Verification items for the finished model (mm, model axes). A direction names the side the tool comes from. Coordinates: 2 decimals unless noted, no trailing zeros. Order: outer loops, then holes, each group sorted by start corner. A loop starts at its lowest first (then second) coordinate and runs counter-clockwise, first axis right, second up. Notation, with made-up numbers: (-17.5, -7) -> (4.5, -7) arc R35 ccw to (4.5, 32) -> close; hole circle Ø3 at (-24.5, -25.5). An arc over 180 degrees is marked (long way). Write item = value, one per line. Start each with the question number.
1. Cross-section at C-C on x = 7. Record the cut outline in (y, z).
2. Cross-section at B-B on z = 12. Record the cut outline in (x, y), plus the area to 3 significant figures.
3. Go/stop test with flat-tipped pins: P1, Ø6.5, axis at x = -1.5, z = 11, coming from the -Y side; P2, Ø6.5, axis at x = -3.5, z = 8, coming from the +Y side; P3, Ø1.5, axis at x = 6, z = 2, coming from the -Y side. Record where each tip stops, or that it passes through.
4. Set-up check for faces 1 (the flat face through (22.458, 14.516, 10.393)), 2 (the flat face through (-12.31, 0, 10)): record each of +Z, -Z, +X, -X, +Y, -Y from which the full face is reachable in a straight line by a thin tool's end or side.
5. Cross-section at D-D on y = 21. Record the cut outline in (x, z).
6. Cross-section at A-A on y = 1. Record the cut outline in (x, z), plus the area to 3 significant figures.
7. Thickness scan on line 1 along X through (y, z) = (3.5, 7.75); line 2 along X through (y, z) = (2, 14); line 3 along Y through (x, z) = (1, 9). Record the ranges inside material, lowest first. Write a range as from..to.
8. Release check for a two-part mould opening along Y. For faces 3 (the flat face through (12.31, 0, 10)), 4 (the flat face through (-23.8, 12.19, 10.39)), 5 (the flat face through (1, 12, 21.082)), 6 (the flat face through (1.342, -26.707, 10.393)) record: +Y half, -Y half, draft (parallel to the pull), parting line (faces both ways), or undercut.
from build123d import *

# Parameters (mm, degrees)
F0_W     = 24.619864
F0_H     = 23.054572
F1_DEPTH = 21.082


with BuildPart() as f1:
    # F0 (on Top) → F1 (new body)
    with BuildSketch(Plane.XY):
        Polygon((-3.977364, 53.318289), (-44.18631, -30.103643), (48.163675, -23.214646), align=None)
        Rectangle(F0_W, F0_H, mode=Mode.SUBTRACT)
    extrude(amount=F1_DEPTH)


solid = f1.part
Worked out:
q1.outline = (-26.29, 0) -> (-11.53, 0) -> (-11.53, 21.08) -> (-26.29, 21.08) -> close; (11.53, 0) -> (37.21, 0) -> (37.21, 21.08) -> (11.53, 21.08) -> close
q2.outline = (-44.19, -30.1) -> (48.16, -23.21) -> (-3.98, 53.32) -> close; hole (-12.31, -11.53) -> (12.31, -11.53) -> (12.31, 11.53) -> (-12.31, 11.53) -> close
q2.area = 3,150 mm²
q3.P1 = -27.16
q3.P2 = 53.32
q3.P3 = -26.42
q4.face_1 = +Z, -Z, +X, +Y
q4.face_2 = +Z, -Z
q5.outline = (-19.55, 0) -> (18.04, 0) -> (18.04, 21.08) -> (-19.55, 21.08) -> close
q6.outline = (-29.19, 0) -> (-12.31, 0) -> (-12.31, 21.08) -> (-29.19, 21.08) -> close; (12.31, 0) -> (31.67, 0) -> (31.67, 21.08) -> (12.31, 21.08) -> close
q6.area = 764 mm²
q7.line_1 = -27.99..-12.31, 12.31..29.96
q7.line_2 = -28.71..-12.31, 12.31..30.99
q7.line_3 = -26.73..-11.53, 11.53..46.01
q8.face_3 = undercut
q8.face_4 = +Y half
q8.face_5 = draft
q8.face_6 = -Y half
